```python
from build123d import *

# Parameters (mm, degrees)
SKETCH1_R           = 15
BOSS_EXTRUDE1_DEPTH = 40
SKETCH2_R           = 4
CUT_EXTRUDE1_DEPTH  = 7
SKETCH6_W           = 2.8
SKETCH6_H           = 1
SKETCH6_W_2         = 1
SKETCH6_H_2         = 2.8
CUT_EXTRUDE4_DEPTH  = 30
SKETCH7_R           = 9.5
CUT_EXTRUDE5_DEPTH  = 3
CUT_EXTRUDE6_REACH  = 44.65
SKETCH8_R           = 1.05
SKETCH9_R           = 3.39912378
BOSS_EXTRUDE2_DEPTH = 4
SKETCH10_R          = 2
CUT_EXTRUDE7_DEPTH  = 4
CUT_EXTRUDE9_START  = -35
SKETCH13_R          = 15
CUT_EXTRUDE9_DEPTH  = 35


with BuildPart() as part:
    # Sketch1 → Boss-Extrude1 (new body)
    with BuildSketch(Plane(origin=(0, 0, 0), x_dir=(1, 0, 0), z_dir=(0, 1, 0))):
        with Locations(Location((0, 0, 0), (0, 0, 270))):
            Circle(SKETCH1_R)
    extrude(amount=BOSS_EXTRUDE1_DEPTH)

    # Sketch2 → Cut-Extrude1 (cut)
    with BuildSketch(Plane(origin=(0, 40, 0), x_dir=(1, 0, 0), z_dir=(0, 1, 0))):
        with Locations(Location((0, 6, 0), (0, 0, 270))):
            Circle(SKETCH2_R)
        with Locations(Location((6, 0, 0), (0, 0, 270))):
            Circle(SKETCH2_R)
        with Locations(Location((0, -6, 0), (0, 0, 270))):
            Circle(SKETCH2_R)
        with Locations(Location((-6, 0, 0), (0, 0, 270))):
            Circle(SKETCH2_R)
    extrude(amount=-CUT_EXTRUDE1_DEPTH, mode=Mode.SUBTRACT)

    # Sketch6 → Cut-Extrude4 (cut)
    with BuildSketch(Plane(origin=(0, 33, 0), x_dir=(1, 0, 0), z_dir=(0, 1, 0))):
        with Locations((0, -6)):
            Rectangle(SKETCH6_W, SKETCH6_H)
        with Locations((6, 0)):
            Rectangle(SKETCH6_W_2, SKETCH6_H_2)
        with Locations((-6, 0)):
            Rectangle(SKETCH6_W_2, SKETCH6_H_2)
        with Locations((0, 6)):
            Rectangle(SKETCH6_W, SKETCH6_H)
    extrude(amount=-CUT_EXTRUDE4_DEPTH, mode=Mode.SUBTRACT)

    # Sketch7 → Cut-Extrude5 (cut)
    with BuildSketch(Plane.XZ):
        with Locations(Location((0, 0, 0), (0, 0, 270))):
            Circle(SKETCH7_R)
    extrude(amount=-CUT_EXTRUDE5_DEPTH, mode=Mode.SUBTRACT)

    # Sketch8 → Cut-Extrude6 (cut, up to next)
    with BuildSketch(Plane.XZ.offset(-3), mode=Mode.PRIVATE) as cut_extrude6_sk1:
        with Locations(Location((0, 0, 0), (0, 0, 270))):
            Circle(SKETCH8_R)
    cut_extrude6_tool1 = extrude(cut_extrude6_sk1.sketch, amount=-CUT_EXTRUDE6_REACH, mode=Mode.PRIVATE) & part.part
    add(cut_extrude6_tool1.solids().sort_by_distance((0, 3, 0))[0], mode=Mode.SUBTRACT)

    # Sketch9 → Boss-Extrude2 (add)
    with BuildSketch(Plane.XZ.offset(-3)):
        with Locations(Location((0, 0, 0), (0, 0, 270))):
            Circle(SKETCH9_R)
    extrude(amount=BOSS_EXTRUDE2_DEPTH)

    # Sketch10 → Cut-Extrude7 (cut)
    with BuildSketch(Plane.XZ.offset(1)):
        with Locations(Location((0, 0, 0), (0, 0, 270))):
            Circle(SKETCH10_R)
    extrude(amount=-CUT_EXTRUDE7_DEPTH, mode=Mode.SUBTRACT)

    # Sketch13 → Cut-Extrude9 (cut)
    with BuildSketch(Plane(origin=(0, 40, 0), x_dir=(1, 0, 0), z_dir=(0, 1, 0)).offset(CUT_EXTRUDE9_START)):
        with Locations(Location((0, 0, 0), (0, 0, 270))):
            Circle(SKETCH13_R)
        Polygon((8.693004096, 4), (13.871626361, 0.715633025), (9.540851678, -2.621495041), (4, -8.693004096), (0.715633025, -13.871626361), (-2.621495041, -9.540851678), (-8.693004096, -4), (-13.871626361, -0.715633025), (-9.540851678, 2.621495041), (-4, 8.693004096), (-0.715633025, 13.871626361), (2.621495041, 9.540851678), align=None, mode=Mode.SUBTRACT)
    extrude(amount=CUT_EXTRUDE9_DEPTH, mode=Mode.SUBTRACT)


solid = part.part
```
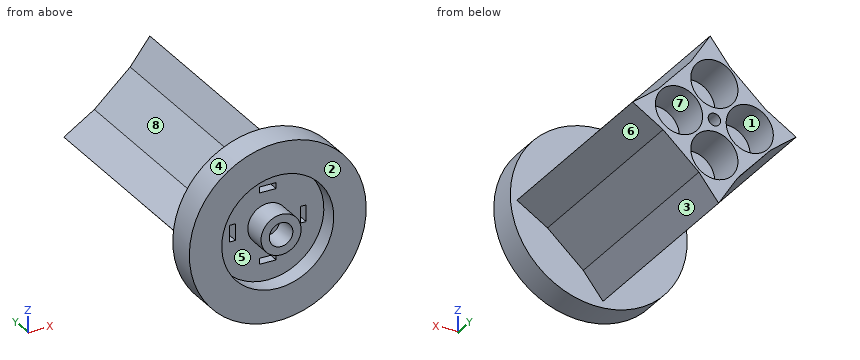
The model under review builds one solid part; all positions refer to its coordinate system, in mm. Face numbers are marked on the shaded views. A direction names the side the tool comes from. Give positions to 0.01 mm unless a question says otherwise; leave off trailing zeros. Write each loop counter-clockwise with the first axis right and the second up, starting at its lowest first coordinate (ties: lowest second). Pieces come first, ordered by that corner, then holes. Notation, with made-up numbers: (54.5, 24) -> (100.5, 24) arc R24 ccw to (100.5, 61) -> close; hole circle Ø4 at (51, -17). An arc over 180 degrees is marked (long way). Put each result on its own line as item: value.
(1) We need section C-C, the plane z = 6. Give the boundary of the cut face in (x, y), and give its area (3 significant figures).
Results are:
outline: (-13.75, 0) -> (-7.37, 0) -> (-7.37, 3) -> (-1.4, 3) -> (-1.4, 33) -> (-4, 33) -> (-4, 40) -> (-6.5, 40) -> (-6.5, 5) -> (-13.75, 5) -> close; (1.4, 3) -> (7.37, 3) -> (7.37, 0) -> (13.75, 0) -> (13.75, 5) -> (6.46, 5) -> (6.46, 40) -> (4, 40) -> (4, 33) -> (1.4, 33) -> close
area: 407 mm²
(2) We need section B-B, the plane x = 6. Give the boundary of the cut face in (y, z).
Results are:
outline: (0, -13.75) -> (5, -13.75) -> (5, -6.46) -> (40, -6.46) -> (40, -4) -> (33, -4) -> (33, -1.4) -> (3, -1.4) -> (3, -7.37) -> (0, -7.37) -> close; (0, 7.37) -> (3, 7.37) -> (3, 1.4) -> (33, 1.4) -> (33, 4) -> (40, 4) -> (40, 6.5) -> (5, 6.5) -> (5, 13.75) -> (0, 13.75) -> close
(3) The part is to be moulded in two halves that separate along Z. For the marked faces 1, 2 and 3, say which applies: pulls with the +Z half, pulls with the -Z half, needs draft (parallel to the pull), parting line crosses it, or undercut.
Results are:
face 1: undercut
face 2: needs draft
face 3: pulls with the -Z half
(4) We need section D-D, the plane y = 24. State how many separate pieces and enclosed holes the cut face has, and give its area (3 significant figures).
Results are:
separate pieces: 1
enclosed holes: 5
area: 315 mm²
(5) We need section A-A, the plane y = 4.5. Give the boundary of the cut face in (x, z).
Results are:
outline: circle Ø30 at (0, 0); hole (-6.5, -1.4) -> (-5.5, -1.4) -> (-5.5, 1.4) -> (-6.5, 1.4) -> close; hole (-1.4, -6.5) -> (1.4, -6.5) -> (1.4, -5.5) -> (-1.4, -5.5) -> close; hole (-1.4, 5.5) -> (1.4, 5.5) -> (1.4, 6.5) -> (-1.4, 6.5) -> close; hole circle Ø2.1 at (0, 0); hole (5.5, -1.4) -> (6.5, -1.4) -> (6.5, 1.4) -> (5.5, 1.4) -> close
(6) To check wall thickness, follow probe 1 along X at (y, z) = (1.5, 0); probe 2 along Z at (x, y) = (0.75, 7); probe 3 along Y at (x, z) = (-9, 1.5). State the ranges of each line that lie inside material, in increasing order. Write a range as from..to.
Results are:
probe 1: -15..-9.5, -3.4..-2, 2..3.4, 9.5..15
probe 2: -11.97..-6.5, -5.5..-0.73, 0.73..5.5, 6.5..13.82
probe 3: 3..33
(7) For pin 1 Ø3 at (x, y) = (-0.5, 25.5) entering from -Z; pin 2 Ø1 at (y, z) = (29, -2) entering from +X; pin 3 Ø0.5 at (x, y) = (6, 13.5) entering from +Z, all flat-tipped, find the tip position at first contact; note any pin that passes through.
Results are:
pin 1: z = -13.87
pin 2: x = 12.63
pin 3: z = 6.78
(8) Tool access review of the marked faces 4, 5, 6, 7 and 8: name each direction out of +Z, -Z, +X, -X, +Y, -Y from which nothing blocks a thin tool from reaching the whole face with its end or side.
Results are:
face 4: +Y, -Y
face 5: -Y
face 6: -Z, +X, +Y
face 7: +Y
face 8: +Z, -X, +Y
